Source: CAD feature listing. Evaluate the final solid. Frame: model axes, mm. Face numbers are marked on the shaded views. A direction names the side the tool comes from. Round coordinates to 2 decimals unless told otherwise and drop trailing zeros. Order: outer loops, then holes, each group sorted by start corner. A loop starts at its lowest first (then second) coordinate and runs counter-clockwise, first axis right, second up. Notation, with made-up numbers: M 70.5,22.5 L 85.5,22.5 A18 cw 85.5,41.5 Z; hole C -22,-33.5 d11. An arc over 180 degrees is marked long. Answer as CSV lines item,"result". Start each with the question number.
Item 1: Section query C-C on y = 48. Return the cut outline in (x, z).
Item 2: Line query: line 1 (X direction, y = 22, z = 0); line 2 (Z direction, x = -1, y = 4.5); line 3 (Y direction, x = -10, z = -3.25). Output: solid intervals per line, ascending. Write a range as [from, to].
Item 3: First-contact query: P1, Ø2, axis at x = 2.5, y = 0.5, coming from the -Z side; P2, Ø11, axis at x = 0, z = 0, coming from the +Y side; P3, Ø4, axis at x = -8.5, z = -9.5, coming from the -Y side; P4, Ø1.5, axis at x = 7, z = 8, coming from the +Y side. Flat tips, straight axial feed; report the tip coordinate or a pass-through.
Item 4: Section query B-B on x = 3. Return the cut outline in (y, z).
Item 5: Section query A-A on z = 0. Return the cut outline in (x, y), plus the area to 3 significant figures.
Item 6: Set-up query: the marked faces 4 and 5. Return all of +Z, -Z, +X, -X, +Y, -Y with unobstructed straight access to the full face (end or side cutting, diameter ignored); none if empty.
Item 7: Pull-direction query (Z, two-part tool) for the marked faces 1, 2 and 3; classes: +Z half, -Z half, draft (parallel to the pull), parting line (faces both ways), or undercut.
Item 8: Section query D-D on y = 26. Return the cut outline in (x, z), plus the area to 3 significant figures.
from build123d import *

# Parameters (mm, degrees)
SKETCH1_R           = 12.5
BOSS_EXTRUDE1_DEPTH = 46
SKETCH2_R           = 8.375
BOSS_EXTRUDE2_DEPTH = 4
SKETCH3_R           = 10
BOSS_EXTRUDE4_DEPTH = 7.6
SKETCH4_R           = 8.5
BOSS_EXTRUDE5_DEPTH = 9
SKETCH5_R           = 5
CUT_EXTRUDE1_DEPTH  = 66.048136022
SKETCH6_R           = 7
CUT_EXTRUDE2_DEPTH  = 66.048136022


with BuildPart() as part:
    # Sketch1 → Boss-Extrude1 (new body)
    with BuildSketch(Plane(origin=(0, 0, 0), x_dir=(1, 0, 0), z_dir=(0, 1, 0))):
        with Locations(Location((0, 0, 0), (0, 0, 270))):
            Circle(SKETCH1_R)
    extrude(amount=BOSS_EXTRUDE1_DEPTH)

    # Sketch2 → Boss-Extrude2 (add)
    with BuildSketch(Plane.XZ):
        with Locations(Location((0, 0, 0), (0, 0, 270))):
            Circle(SKETCH2_R)
    extrude(amount=BOSS_EXTRUDE2_DEPTH)

    # Sketch3 → Boss-Extrude4 (add)
    with BuildSketch(Plane(origin=(0, 46, 0), x_dir=(1, 0, 0), z_dir=(0, 1, 0))):
        with Locations(Location((0, 0, 0), (0, 0, 90))):
            Circle(SKETCH3_R)
    extrude(amount=BOSS_EXTRUDE4_DEPTH)

    # Sketch4 → Boss-Extrude5 (add)
    with BuildSketch(Plane.XZ):
        with Locations(Location((0, 0, 0), (0, 0, 90))):
            Circle(SKETCH4_R)
    extrude(amount=BOSS_EXTRUDE5_DEPTH)

    # Sketch5 → Cut-Extrude1 (cut, through all)
    with BuildSketch(Plane(origin=(0, 53.6, 0), x_dir=(1, 0, 0), z_dir=(0, 1, 0))):
        with Locations(Location((0, 0, 0), (0, 0, 270))):
            Circle(SKETCH5_R)
    extrude(amount=-CUT_EXTRUDE1_DEPTH, mode=Mode.SUBTRACT)

    # Sketch6 → Cut-Extrude2 (cut, through all)
    with BuildSketch(Plane(origin=(0, 53.6, 0), x_dir=(1, 0, 0), z_dir=(0, 1, 0))):
        with Locations(Location((0, 0, 0), (0, 0, 270))):
            Circle(SKETCH6_R)
    extrude(amount=-CUT_EXTRUDE2_DEPTH, mode=Mode.SUBTRACT)


solid = part.part
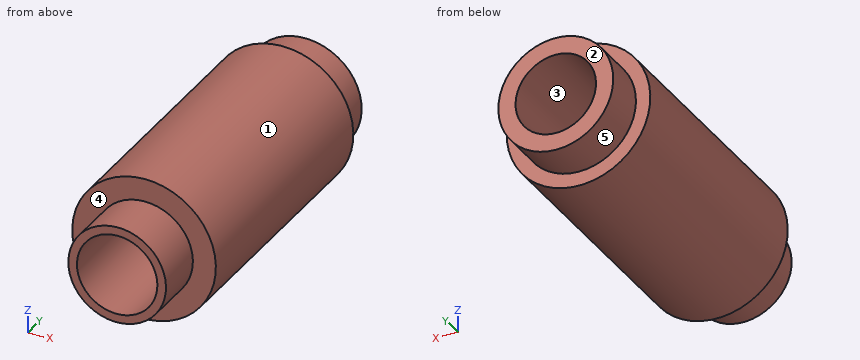
Results:
1,outline,"C 0,0 d20; hole C 0,0 d14"
2,line 1,"[-12.5, -7], [7, 12.5]"
2,line 2,"[-12.46, -6.93], [6.93, 12.46]"
2,line 3,"[0, 46]"
3,P1,"z = -12.41"
3,P2,"through"
3,P3,"y = 0"
3,P4,"y = 53.6"
4,outline,"M -9,-7.95 L 0,-7.95 L 0,-12.13 L 46,-12.13 L 46,-9.54 L 53.6,-9.54 L 53.6,-6.32 L -9,-6.32 Z; M -9,6.32 L 53.6,6.32 L 53.6,9.54 L 46,9.54 L 46,12.13 L 0,12.13 L 0,7.95 L -9,7.95 Z"
5,outline,"M -12.5,0 L -8.5,0 L -8.5,-9 L -7,-9 L -7,53.6 L -10,53.6 L -10,46 L -12.5,46 Z; M 7,-9 L 8.5,-9 L 8.5,0 L 12.5,0 L 12.5,46 L 10,46 L 10,53.6 L 7,53.6 Z"
5,area,"579 mm^2"
6,face 4,"-Y"
6,face 5,"+Y"
7,face 1,"parting line"
7,face 2,"draft"
7,face 3,"undercut"
8,outline,"C 0,0 d25; hole C 0,0 d14"
8,area,"337 mm^2"
